Source: CAD feature listing. Evaluate the final solid. Frame: model axes, mm. A direction names the side the tool comes from. Coordinates: 2 decimals unless noted, no trailing zeros. Write each loop counter-clockwise with the first axis right and the second up, starting at its lowest first coordinate (ties: lowest second). Pieces come first, ordered by that corner, then holes. Notation, with made-up numbers: M 40,-30 L 50,-30 A8 cw 50,-25 Z; hole C 62,-31 d8. An arc over 180 degrees is marked long. One line per item, written item: value. Start each with the question number.
Item 1: Cut plane D-D, the plane z = 15. Output: boundary loops of the cut face in (x, y).
Item 2: Set-up query: faces 1 (the flat face through (-26.178, -26, 9)), 2 (the flat face through (21.822, 13, 8)). Return all of +Z, -Z, +X, -X, +Y, -Y with unobstructed straight access to the full face (end or side cutting, diameter ignored); none if empty.
Item 3: Pin query (flat end, axial travel): P1, Ø4, axis at x = 9.5, y = 34, coming from the -Z side; P2, Ø3, axis at x = -7.5, y = -25, coming from the +Z side. Return the tip coordinate at first contact, or that it passes through.
Item 4: Ray query, L1, parallel to Y at x = -13, z = 5.5; L2, parallel to X at y = -15.5, z = 12.25; L3, parallel to X at y = 51.5, z = 3.75. Return the intervals inside material, ascending. Write a range as from..to.
Item 5: Cut plane A-A, the plane z = 6. Output: boundary loops of the cut face in (x, y), then the cut area to 3 significant figures.
Item 6: Cut plane B-B, the plane y = 45. Output: boundary loops of the cut face in (x, z).
Item 7: Cut plane C-C, the plane x = -27.5. Output: boundary loops of the cut face in (y, z), then the cut area to 4 significant figures.
Item 8: Mould query, pull axis X, two halves, no side actions, for faces 3 (the conical face through (17.66, 51.87, 9.66)), 4 (the cylindrical face through (20.92, 54.804, 8.085)), 5 (the cylindrical face through (-33.32, -29.74, 8.31)), 6 (the flat face through (-6, -30.641, 8)). Classes: released by +X, released by -X, zero draft, split by the parting line, or undercut.
Autodesk Inventor part; units mm, degrees
ref_plane "YZ Plane" through (0, 0, 0) normal (1, 0, 0) x (0, 1, 0)
ref_plane "XZ Plane" through (0, 0, 0) normal (0, 1, 0) x (-1, 0, 0)
ref_plane "XY Plane" through (0, 0, 0) normal (0, 0, 1) x (1, 0, 0)
sketch "Sketch1" plane through (0, 0, 0) normal (0, 0, 1) x (1, 0, 0)
  line L0 (-34.1779, 55.6594) -> (21.8221, 55.6594)
  line L1 (21.8221, 55.6594) -> (21.8221, -30.6406)
  line L2 (21.8221, -30.6406) -> (-34.1779, -30.6406)
  line L3 (-34.1779, -30.6406) -> (-34.1779, 55.6594)
  point P0 (0, 0)
  dimension "d0" = 56
  dimension "d1" = 86.3
extrude "Extrusion1" add sketch "Sketch1" along normal blind 2
sketch "Sketch2" plane through (0, 0, 2) normal (0, 0, 1) x (1, 0, 0)
  line L0 (-34.1779, 55.6594) -> (21.8221, 55.6594)
  line L1 (21.8221, 55.6594) -> (21.8221, -30.6406)
  line L2 (21.8221, -30.6406) -> (-34.1779, -30.6406)
  line L3 (-34.1779, -30.6406) -> (-34.1779, 55.6594)
  line L4 (-32.1779, 53.6594) -> (19.8221, 53.6594)
  line L5 (19.8221, 53.6594) -> (19.8221, -28.6406)
  line L6 (19.8221, -28.6406) -> (-32.1779, -28.6406)
  line L7 (-32.1779, -28.6406) -> (-32.1779, 53.6594)
  point P0 (0, 0)
  dimension "d4" = 2
  dimension "d5" = 2
  dimension "d6" = 2
  dimension "d7" = 2
extrude "Extrusion2" add sketch "Sketch2" along normal blind 14.4
sketch "Sketch3" plane through (0, 0, 2) normal (0, 0, 1) x (1, 0, 0)
  line L0 (-34.1779, 55.6594) -> (-26.1779, 55.6594)
  line L1 (-26.1779, 55.6594) -> (-26.1779, 47.6594)
  line L2 (-26.1779, 47.6594) -> (-34.1779, 47.6594)
  line L3 (-34.1779, 47.6594) -> (-34.1779, 55.6594)
  line L4 (21.8221, 55.6594) -> (13.8221, 55.6594)
  line L5 (13.8221, 55.6594) -> (13.8221, 47.6594)
  line L6 (13.8221, 47.6594) -> (21.8221, 47.6594)
  line L7 (21.8221, 47.6594) -> (21.8221, 55.6594)
  line L8 (-34.1779, -30.6406) -> (-26.1779, -30.6406)
  line L9 (-26.1779, -30.6406) -> (-26.1779, -22.6406)
  line L10 (-26.1779, -22.6406) -> (-34.1779, -22.6406)
  line L11 (-34.1779, -22.6406) -> (-34.1779, -30.6406)
  line L12 (21.8221, -30.6406) -> (13.8221, -30.6406)
  line L13 (13.8221, -30.6406) -> (13.8221, -22.6406)
  line L14 (13.8221, -22.6406) -> (21.8221, -22.6406)
  line L15 (21.8221, -22.6406) -> (21.8221, -30.6406)
  line L16 (-34.1779, -30.6406) -> (21.8221, -30.6406)
  point P0 (0, 0)
  dimension "d10" = 8
  dimension "d11" = 8
  dimension "d12" = 8
  dimension "d13" = 8
  dimension "d14" = 8
  dimension "d15" = 8
  dimension "d16" = 8
  dimension "d17" = 8
extrude "Extrusion3" add sketch "Sketch3" along normal blind 14.4
sketch "Sketch4" plane through (0, 0, 16.4) normal (0, 0, 1) x (1, 0, 0)
  line L0 (-26.1779, -22.6406) -> (-32.1779, -22.6406)
  line L1 (19.8221, -22.6406) -> (13.8221, -22.6406)
  line L2 (21.8221, 55.6594) -> (21.8221, -30.6406)
  line L3 (21.8221, 55.6594) -> (-34.1779, 55.6594)
  line L4 (-34.1779, -30.6406) -> (-34.1779, 55.6594)
  point P0 (0, 0)
  point P1 (-30.1779, 51.6594)
  point P2 (17.8221, 51.6594)
  point P3 (-30.5754, -26.6406)
  point P4 (17.8221, -26.6406)
  dimension "d20" = 4
  dimension "d21" = 4
  dimension "d22" = 4
  dimension "d23" = 4
  dimension "d24" = 4
  dimension "d25" = 4
  dimension "d26" = 4
hole "Hole1" at (-30.1779, 51.6594, 16.4) at (17.8221, 51.6594, 16.4) at (-30.5754, -26.6406, 16.4) at (17.8221, -26.6406, 16.4) direction (0, 0, -1) diameter 3 depth 6 tip angle 118
fillet "Fillet1" radius 3 4 edges at (-34.1779, 55.6594, 8.2) (21.8221, 55.6594, 8.2) (-34.1779, -30.6406, 8.2) (21.8221, -30.6406, 8.2)
sketch "Sketch5" plane through (0, 0, 2) normal (0, 0, 1) x (1, 0, 0)
  line L0 (-32.1779, 47.6594) -> (19.8221, 47.6594)
  line L1 (19.8221, 47.6594) -> (19.8221, 43.3594)
  line L2 (19.8221, 43.3594) -> (-32.1779, 43.3594)
  line L3 (-32.1779, 43.3594) -> (-32.1779, 47.6594)
  line L4 (19.8221, 47.6594) -> (19.8221, -22.6406)
  line L5 (-32.1779, -22.6406) -> (19.8221, -22.6406)
  line L6 (19.8221, -22.6406) -> (19.8221, -18.3406)
  line L7 (19.8221, -18.3406) -> (-32.1779, -18.3406)
  line L8 (-32.1779, -18.3406) -> (-32.1779, -22.6406)
  point P0 (0, 0)
  dimension "d35" = 4.3
  dimension "d36" = 4.3
extrude "Extrusion4" add sketch "Sketch5" along normal blind 2.5
properties part number "base v2"
From the geometry:
1. outline: M -34.18,-27.64 A3 ccw -31.18,-30.64 L 18.82,-30.64 A3 ccw 21.82,-27.64 L 21.82,52.66 A3 ccw 18.82,55.66 L -31.18,55.66 A3 ccw -34.18,52.66 Z; hole M -32.18,-22.64 L -26.18,-22.64 L -26.18,-28.64 L 13.82,-28.64 L 13.82,-22.64 L 19.82,-22.64 L 19.82,47.66 L 13.82,47.66 L 13.82,53.66 L -26.18,53.66 L -26.18,47.66 L -32.18,47.66 Z; hole C -30.58,-26.64 d3; hole C -30.18,51.66 d3; hole C 17.82,-26.64 d3; hole C 17.82,51.66 d3
2. face 1: +Z
2. face 2: +Z, -Z, +X, +Y, -Y
3. P1: stops at z = 0
3. P2: stops at z = 2
4. L1: y = -30.64..-28.64, 53.66..55.66
4. L2: x = -34.18..-32.18, 19.82..21.82
4. L3: x = -34.18..-26.18, 13.82..21.82
5. outline: M -34.18,-27.64 A3 ccw -31.18,-30.64 L 18.82,-30.64 A3 ccw 21.82,-27.64 L 21.82,52.66 A3 ccw 18.82,55.66 L -31.18,55.66 A3 ccw -34.18,52.66 Z; hole M -32.18,-22.64 L -26.18,-22.64 L -26.18,-28.64 L 13.82,-28.64 L 13.82,-22.64 L 19.82,-22.64 L 19.82,47.66 L 13.82,47.66 L 13.82,53.66 L -26.18,53.66 L -26.18,47.66 L -32.18,47.66 Z
5. area: 689 mm²
6. outline: M -34.18,0 L 21.82,0 L 21.82,16.4 L 19.82,16.4 L 19.82,4.5 L -32.18,4.5 L -32.18,16.4 L -34.18,16.4 Z
7. outline: M -30.64,0 L 55.66,0 L 55.66,16.4 L 47.66,16.4 L 47.66,4.5 L 43.36,4.5 L 43.36,2 L -18.34,2 L -18.34,4.5 L -22.64,4.5 L -22.64,16.4 L -30.64,16.4 Z
7. area: 424.5 mm²
8. face 3: undercut
8. face 4: released by +X
8. face 5: released by -X
8. face 6: zero draft
